Part model, mm, in its own coordinate system. A direction names the side the tool comes from. Round coordinates to 2 decimals unless told otherwise and drop trailing zeros. Loops run counter-clockwise (first coordinate to the right, second up) from the corner with the lowest first, then second, coordinate; pieces in that order, holes last. Notation, with made-up numbers: (25, 69.25) -> (49, 69.25) arc R13 cw to (49, 88.25) -> close; hole circle Ø5 at (-38, 70). An arc over 180 degrees is marked (long way). Answer as CSV lines item,"result".
from build123d import *

# Parameters (mm, degrees)
F0_W     = 120
F0_H     = 60
F1_DEPTH = 30
F2_R     = 9
F3_DEPTH = 15


with BuildPart() as f1:
    # F0 (on Front) → F1 (new body, symmetric)
    with BuildSketch(Plane.XZ):
        with Locations((60, 30)):
            Rectangle(F0_W, F0_H)
    extrude(amount=F1_DEPTH, both=True)

    # F2 (on face) → F3 (join)
    with BuildSketch(Plane.XY.offset(60)):
        with Locations((30, 0)):
            Circle(F2_R)
    extrude(amount=F3_DEPTH)


solid = f1.part
Q1. Saw through at A-A, the plane y = 0. Write the cut outline in (x, z), then the cut area to 3 significant figures.
Geometry results:
outline,"(0, 0) -> (120, 0) -> (120, 60) -> (39, 60) -> (39, 75) -> (21, 75) -> (21, 60) -> (0, 60) -> close"
area,"7,470 mm2"
Q2. Saw through at B-B, the plane x = 30. Write the cut outline in (y, z), then the cut area to 3 significant figures.
Geometry results:
outline,"(-30, 0) -> (30, 0) -> (30, 60) -> (9, 60) -> (9, 75) -> (-9, 75) -> (-9, 60) -> (-30, 60) -> close"
area,"3,870 mm2"
Q3. Which spindle directions (+Z, -Z, +X, -X, +Y, -Y) get a long thin tool onto all of the face, cutting with end or side? Do faces 1 (the face through (21, 0, 67)), 2 (the face through (59, 30, 30)). Say none if no direction does.
Geometry results:
face 1,"+Z"
face 2,"+Z, -Z, +X, -X, +Y"
Q4. Saw through at D-D, the plane y = 19.5. Write the cut outline in (x, z), then the cut area to 3 significant figures.
Geometry results:
outline,"(0, 0) -> (120, 0) -> (120, 60) -> (0, 60) -> close"
area,"7,200 mm2"
Q5. Saw through at C-C, the plane x = 78. Write the cut outline in (y, z), then the cut area to 3 significant figures.
Geometry results:
outline,"(-30, 0) -> (30, 0) -> (30, 60) -> (-30, 60) -> close"
area,"3,600 mm2"
Q6. Drill centre line: line 1 along Z through (x, y) = (104.5, 6.5). Where is it in solid material? Low to high.
Geometry results:
line 1,"0 to 60"
Q7. Drop flat-ended pins along their axis: P1, Ø2, axis at x = 71, y = 11.5, coming from the -Z side; P2, Ø2, axis at x = 18.5, y = -22.5, coming from the +Z side. Give the stop position or say it passes through.
Geometry results:
P1,"z = 0"
P2,"z = 60"
